Geometry: see drawing. Coordinates: mm, zero at the bounding-box minimum. Coordinates: 2 decimals unless noted, no trailing zeros. Write each loop counter-clockwise with the first axis right and the second up, starting at its lowest first coordinate (ties: lowest second). Pieces come first, ordered by that corner, then holes. Notation, with made-up numbers: (-33.75, 26) - (8.25, 26) arc R20 cw to (8.25, 57) - close; hole circle Ø2 at (18.5, 57). An arc over 180 degrees is marked (long way). Use a Markdown table: item, result. Add a question column.
Q1. Section query B-B (y = 5). Return the cut outline in (x, z), then the cut area to 3 significant figures.
Q2. Section query C-C (z = 1.2). Return the cut outline in (x, y).
Q3. Section query A-A (x = 4.95). Return the cut outline in (y, z).
Q4. Material intervals for probe 1 along X at (y, z) = (5, 1.5); probe 2 along Y at (x, z) = (4.95, 1.9); probe 3 along Y at (x, z) = (6.25, 4.2), sorted ascending. Write a range as from..to.
Q5. Pin query (flat end, axial travel): P1, Ø3, axis at x = 4.95, y = 5, coming from the -Z side. Return the tip coordinate at first contact, or that it passes through.
Q6. Mould query, pull axis X, two halves, no side actions, for the marked faces 1, 2 and 3. Classes: released by +X, released by -X, zero draft, split by the parting line, or undercut.
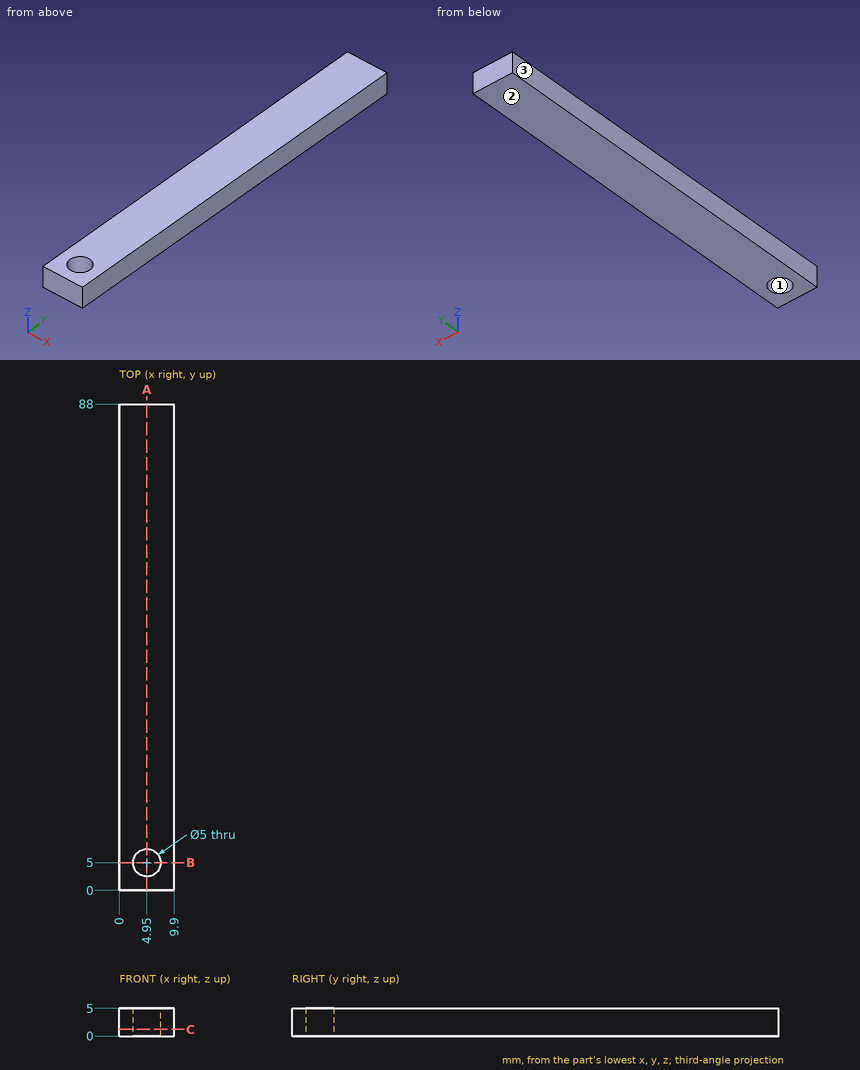
Values follow:
| question | item | result |
|---|---|---|
| 1 | outline | (0, 0) - (2.45, 0) - (2.45, 5) - (0, 5) - close; (7.45, 0) - (9.9, 0) - (9.9, 5) - (7.45, 5) - close |
| 1 | area | 24.5 mm2 |
| 2 | outline | (0, 0) - (9.9, 0) - (9.9, 88) - (0, 88) - close; hole circle Ø5 at (4.95, 5) |
| 3 | outline | (0, 0) - (2.5, 0) - (2.5, 5) - (0, 5) - close; (7.5, 0) - (88, 0) - (88, 5) - (7.5, 5) - close |
| 4 | probe 1 | 0..2.45, 7.45..9.9 |
| 4 | probe 2 | 0..2.5, 7.5..88 |
| 4 | probe 3 | 0..2.86, 7.14..88 |
| 5 | P1 | through |
| 6 | face 1 | undercut |
| 6 | face 2 | zero draft |
| 6 | face 3 | released by -X |
